Source: three-view drawing plus pictorial views. Frame: mm from the lowest corner of the part. A direction names the side the tool comes from. Give positions to 0.01 mm unless a question says otherwise; leave off trailing zeros. Loops run counter-clockwise (first coordinate to the right, second up) from the corner with the lowest first, then second, coordinate; pieces in that order, holes last.
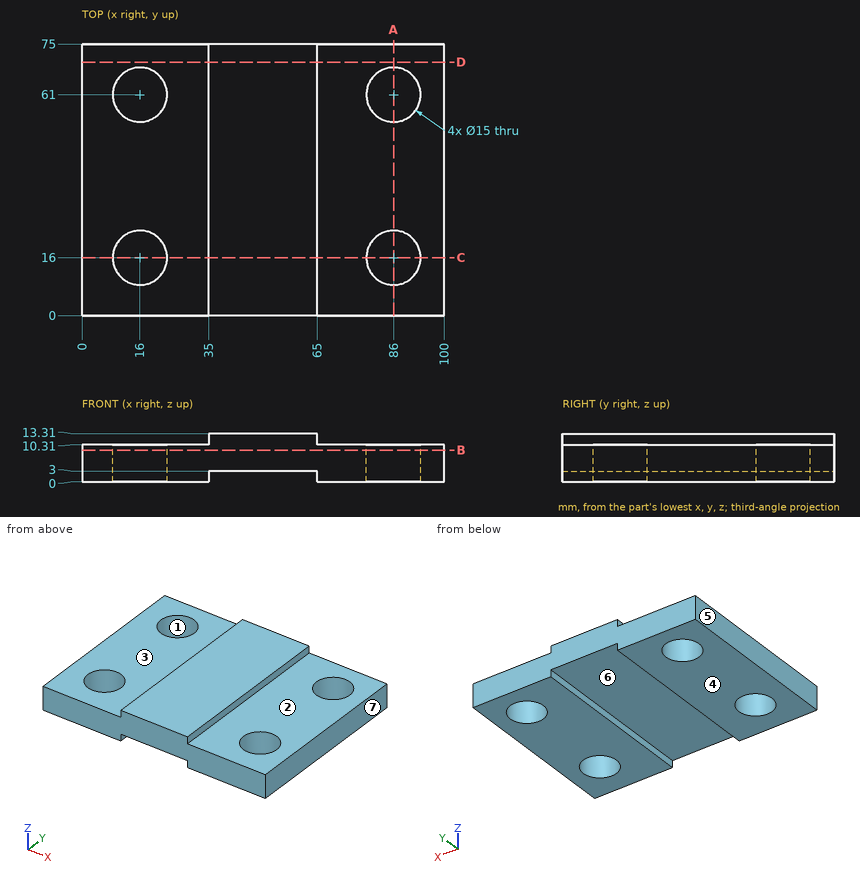
1) Cut plane D-D (y = 70). Return loops of the section in (x, z).
Checks:
outline: (0, 0) - (35, 0) - (35, 3) - (65, 3) - (65, 0) - (100, 0) - (100, 10.31) - (65, 10.31) - (65, 13.31) - (35, 13.31) - (35, 10.31) - (0, 10.31) - close
2) Cut plane C-C (y = 16). Return loops of the section in (x, z), and give its area (3 significant figures).
Checks:
outline: (0, 0) - (8.5, 0) - (8.5, 10.31) - (0, 10.31) - close; (23.5, 0) - (35, 0) - (35, 3) - (65, 3) - (65, 0) - (78.5, 0) - (78.5, 10.31) - (65, 10.31) - (65, 13.31) - (35, 13.31) - (35, 10.31) - (23.5, 10.31) - close; (93.5, 0) - (100, 0) - (100, 10.31) - (93.5, 10.31) - close
area: 722 mm2
3) Contact query for flat-ended pins moving along their axis: P1, Ø3.5, axis at y = 44.5, z = 11.5, coming from the +X side; P2, Ø17.5, axis at x = 78.5, y = 30, coming from the +Z side; P3, Ø15, axis at x = 56, y = 33.5, coming from the -Z side. Output: stop coordinate, or through.
Checks:
P1: stops at x = 100
P2: stops at z = 10.31
P3: stops at z = 3
4) Ray query, probe 1 along Y at (x, z) = (16, 3); probe 2 along X at (y, z) = (61, 2.5); probe 3 along X at (y, z) = (13, 4.75). Return the intervals inside material, ascending.
Checks:
probe 1: y = 0 to 8.5, 23.5 to 53.5, 68.5 to 75
probe 2: x = 0 to 8.5, 23.5 to 35, 65 to 78.5, 93.5 to 100
probe 3: x = 0 to 9.13, 22.87 to 79.13, 92.87 to 100
5) Cut plane B-B (z = 8.75). Return loops of the section in (x, y), and give its area (3 significant figures).
Checks:
outline: (0, 0) - (100, 0) - (100, 75) - (0, 75) - close; hole circle Ø15 at (16, 16); hole circle Ø15 at (16, 61); hole circle Ø15 at (86, 16); hole circle Ø15 at (86, 61)
area: 6,790 mm2
6) Pull-direction query (X, two-part tool) for the marked faces 4, 5, 6 and 7; classes: released by +X, released by -X, zero draft, split by the parting line, or undercut.
Checks:
face 4: zero draft
face 5: released by -X
face 6: undercut
face 7: released by +X
7) Cut plane A-A (x = 86). Return loops of the section in (y, z).
Checks:
outline: (0, 0) - (8.5, 0) - (8.5, 10.31) - (0, 10.31) - close; (23.5, 0) - (53.5, 0) - (53.5, 10.31) - (23.5, 10.31) - close; (68.5, 0) - (75, 0) - (75, 10.31) - (68.5, 10.31) - close
8) Reachability of the marked faces 1, 2 and 3 from +Z, -Z, +X, -X, +Y, -Y: full face, straight path, thin tool, end or side. Return the list, or none.
Checks:
face 1: +Z, -Z
face 2: +Z, +X, +Y, -Y
face 3: +Z, -X, +Y, -Y
